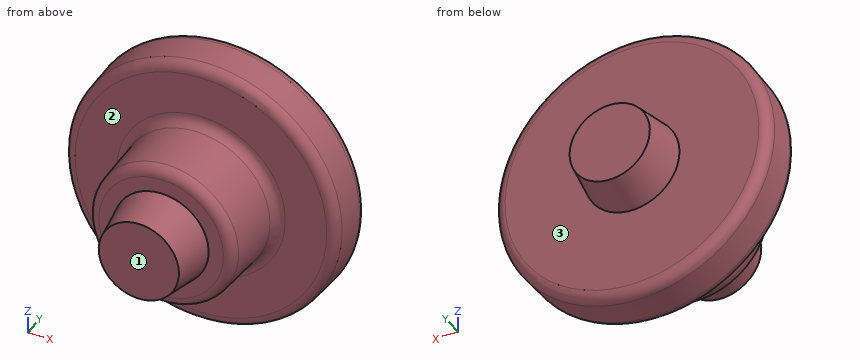
Solid Edge part; units mm, degrees
sketch "Sketch1" plane through (0, 0, 0) normal (1, 0, 0) x (0, 1, 0)
  line L0 (74, 81.0476) -> (74, 0)
  line L1 (44, 80) -> (74, 81.0476)
  line L2 (44, 80) -> (44, 44.0365)
  line L3 (0, 42.5) -> (44, 44.0365)
  line L4 (0, 42.5) -> (0, 0)
  dimension "D1" = 44
  dimension "D2" = 74
revolve "RevolvedProtrusion1" add sketch "Sketch1" angle 360 about axis through (0, 0, 0) along (0, 1, 0)
fillet "Raccordi_grezzo" radius 6 4 edges at (0, 74, 81.0476) (0, 44, 80) (0, 44, 44.0365) (0, 0, 42.5)
sketch "Sketch2" plane through (0, 0, 0) normal (-1, 0, 0) x (0, -1, 0)
  line L0 (0, 0) -> (0, 28)
  line L1 (0, 28) -> (24.6202, 23.6588)
  line L2 (24.6202, 23.6588) -> (24.6202, 0)
revolve "RevolvedProtrusion2" add sketch "Sketch2" angle 360 about axis through (0, -24.6202, 0) along (0, 1, 0)
sketch "Sketch3" plane through (0, 0, 0) normal (-1, 0, 0) x (0, -1, 0)
  line L0 (-74, 0) -> (-74, 28)
  line L1 (-74, 28) -> (-98.6202, 23.6588)
  line L2 (-98.6202, 23.6588) -> (-98.6202, 0)
revolve "RevolvedProtrusion3" add sketch "Sketch3" angle 360 about axis through (0, 98.6202, 0) along (0, -1, 0)
properties material "Acciaio"
Work out the finished part from the listing and answer in its coordinate system (mm). Face numbers are marked on the shaded views. A direction names the side the tool comes from. Coordinates: 2 decimals unless noted, no trailing zeros. Write each loop counter-clockwise with the first axis right and the second up, starting at its lowest first coordinate (ties: lowest second). Pieces come first, ordered by that corner, then holes.
Q1. A cutting plane is placed at A-A, the plane z = 0. Give the vertices of the cut face in (x, y), then the cut area to 3 significant figures.
Q2. Each of these flat-tipped pins is pushed along its axis until it touches: pin 1 Ø4 at (x, y) = (-13, -4) entering from -Z; pin 2 Ø1 at (y, z) = (71.5, 63) entering from +X; pin 3 Ø10 at (x, z) = (34, -27.5) entering from +Y. Where does it stop, or does it pass through?
Q3. A cutting plane is placed at B-B, the plane x = 0. Give the vertices of the cut face in (y, z), then the cut area to 3 significant figures.
Q4. A cutting plane is placed at C-C, the plane y = 15.5. Give the vertices of the cut face in (x, z).
Q5. A cutting plane is placed at D-D, the plane y = 53.5. Give the vertices of the cut face in (x, z), then the cut area to 3 significant figures.
Q6. Which of the six approach directions +Z, -Z, +X, -X, +Y, -Y give full straight-line access (tool end or side, diameter ignored) to the marked faces 1, 2 and 3?
Q7. Find the intervals of material crossed by line 1 (Y direction, x = 30.5, z = -42); line 2 (Y direction, x = 15, z = 30.5); line 3 (Z direction, x = 30, y = 70.5), in increasing order.
Findings below:
1. outline: (-80.83, 67.79) - (-80.2, 49.79) arc R6 ccw to (-74.21, 44) - (-49.83, 44) arc R6 cw to (-43.83, 38.21) - (-42.7, 5.79) arc R6 ccw to (-36.71, 0) - (-28, 0) - (-23.66, -24.62) - (23.66, -24.62) - (28, 0) - (36.71, 0) arc R6 ccw to (42.7, 5.79) - (43.83, 38.21) arc R6 cw to (49.83, 44) - (74.21, 44) arc R6 ccw to (80.2, 49.79) - (80.83, 67.79) arc R6 ccw to (74.83, 74) - (28, 74) - (23.66, 98.62) - (-23.66, 98.62) - (-28, 74) - (-74.83, 74) arc R6 ccw to start
1. area: 11,200 mm2
2. pin 1: stops at z = -25.06
2. pin 2: stops at x = 49.67
2. pin 3: stops at y = 74
3. outline: (-24.62, -23.66) - (0, -28) - (0, -36.71) arc R6 ccw to (5.79, -42.7) - (38.21, -43.83) arc R6 cw to (44, -49.83) - (44, -74.21) arc R6 ccw to (49.79, -80.2) - (67.79, -80.83) arc R6 ccw to (74, -74.83) - (74, -28) - (98.62, -23.66) - (98.62, 23.66) - (74, 28) - (74, 74.83) arc R6 ccw to (67.79, 80.83) - (49.79, 80.2) arc R6 ccw to (44, 74.21) - (44, 49.83) arc R6 cw to (38.21, 43.83) - (5.79, 42.7) arc R6 ccw to (0, 36.71) - (0, 28) - (-24.62, 23.66) - close
3. area: 11,200 mm2
4. outline: circle Ø86.08 at (0, 0)
5. outline: circle Ø160.66 at (0, 0)
5. area: 20,300 mm2
6. face 1: +Z, -Z, +X, -X, -Y
6. face 2: -Y
6. face 3: +Y
7. line 1: y = 44 to 74
7. line 2: y = 0 to 74
7. line 3: z = -74.47 to 74.47
